Model file for the job. Use its own axes, mm. Face numbers are marked on the shaded views. Coordinates: 2 decimals unless noted, no trailing zeros. Order: outer loops, then holes, each group sorted by start corner. A loop starts at its lowest first (then second) coordinate and runs counter-clockwise, first axis right, second up. Notation, with made-up numbers: M 69.5,53 L 111.5,53 A19 cw 111.5,69 Z; hole C -3,0.5 d7. An arc over 180 degrees is marked long. Return JSON: item names as keys, results as strings.
```python
from build123d import *

# Parameters (mm, degrees)
CORTAR_EXTRUIR1_DEPTH = 50
CROQUIS4_R            = 1.5
CORTAR_EXTRUIR2_DEPTH = 20


with BuildPart() as part:
    # Croquis1 → Revolución1 (revolve)
    with BuildSketch(Plane(origin=(0, 0, 0), x_dir=(1, 0, 0), z_dir=(0, 1, 0))):
        with BuildLine():
            Line((-10, 0), (-18, 0))
            Line((-18, 0), (-18, 11.630777084))
            Line((-18, 11.630777084), (1.574675275, 11.630777084))
            Line((1.574675275, 11.630777084), (1.574675275, 9.875241657))
            ThreePointArc((1.574675275, 9.875241657), (-6.490502571, 7.607455315), (-10, 0))
        make_face()
    revolve(axis=Axis((-10, 0, 0), (-1, 0, 0)))

    # Croquis3 → Cortar-Extruir1 (cut)
    with BuildSketch(Plane(origin=(1.574675275, 0, 0), x_dir=(0, 0, -1), z_dir=(1, 0, 0))):
        Polygon((0, 0), (0, -16.586651977), (12.985125339, -16.586651977), (12.985125339, 15.917262398), (0, 15.917262398), align=None)
    extrude(amount=-CORTAR_EXTRUIR1_DEPTH, mode=Mode.SUBTRACT)

    # Croquis4 → Cortar-Extruir2 (cut)
    with BuildSketch(Plane(origin=(0, 0, 0), x_dir=(-1, 0, 0), z_dir=(0, 0, -1))):
        with Locations((13.917030973, 0)):
            Circle(CROQUIS4_R)
    extrude(amount=-CORTAR_EXTRUIR2_DEPTH, mode=Mode.SUBTRACT)


solid = part.part
```
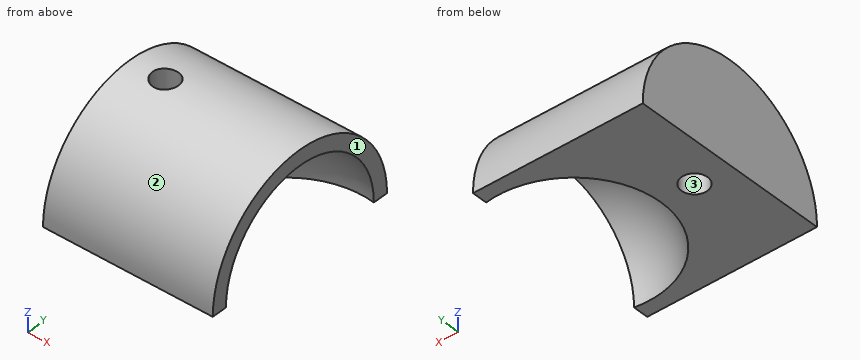
Item 1: Wall check: line 1 (Y direction, x = 0.5, z = 1); line 2 (X direction, y = 0, z = 5); line 3 (Y direction, x = -6.75, z = 6). Give the ranges that are in metal, low to high.
Check result:
{"line 1": "y = -11.59 to -9.94, 9.94 to 11.59", "line 2": "x = -18 to -15.42, -12.42 to -8.66", "line 3": "y = -9.96 to -4.29, 4.29 to 9.96"}
Item 2: Drop flat-ended pins along their axis: pin 1 Ø1.5 at (x, y) = (-11.5, 4) entering from +Z; pin 2 Ø6 at (x, y) = (-14.5, -7.5) entering from +Z. Give the stop position or say it passes through.
Check result:
{"pin 1": "stops at z = 11.17", "pin 2": "stops at z = 10.72"}
Item 3: Pull direction Y, two halves, no side cores. Call the marked faces 1, 2 and 3: +Y half, -Y half, draft (parallel to the pull), parting line (faces both ways), or undercut.
Check result:
{"face 1": "draft", "face 2": "parting line", "face 3": "undercut"}
Item 4: Saw through at B-B (z = 1.5). Write the cut outline in (x, y), and give its area (3 significant figures).
Check result:
{"outline": "M -18,-11.53 L 1.57,-11.53 L 1.57,-9.76 A9.89 cw long 1.57,9.76 L 1.57,11.53 L -18,11.53 Z; hole C -13.92,0 d3", "area": "260 mm2"}
Item 5: Saw through at D-D (x = 0.75). Write the cut outline in (y, z), and give its area (3 significant figures).
Check result:
{"outline": "M -11.63,0 L -9.97,0 A9.97 cw 9.97,0 L 11.63,0 A11.63 ccw Z", "area": "56.3 mm2"}
Item 6: Saw through at C-C (y = -3.5). Write the cut outline in (x, z) (1 decimal), and give its area (3 significant figures).
Check result:
{"outline": "M -18,0 L -9.4,0 A9.4 cw 1.6,9.2 L 1.6,11.1 L -18,11.1 Z", "area": "134 mm2"}
Item 7: Saw through at A-A (y = 0). Write the cut outline in (x, z), and give its area (3 significant figures).
Check result:
{"outline": "M -18,0 L -15.42,0 L -15.42,11.63 L -18,11.63 Z; M -12.42,0 L -10,0 A10 cw 1.57,9.88 L 1.57,11.63 L -12.42,11.63 Z", "area": "98.6 mm2"}
